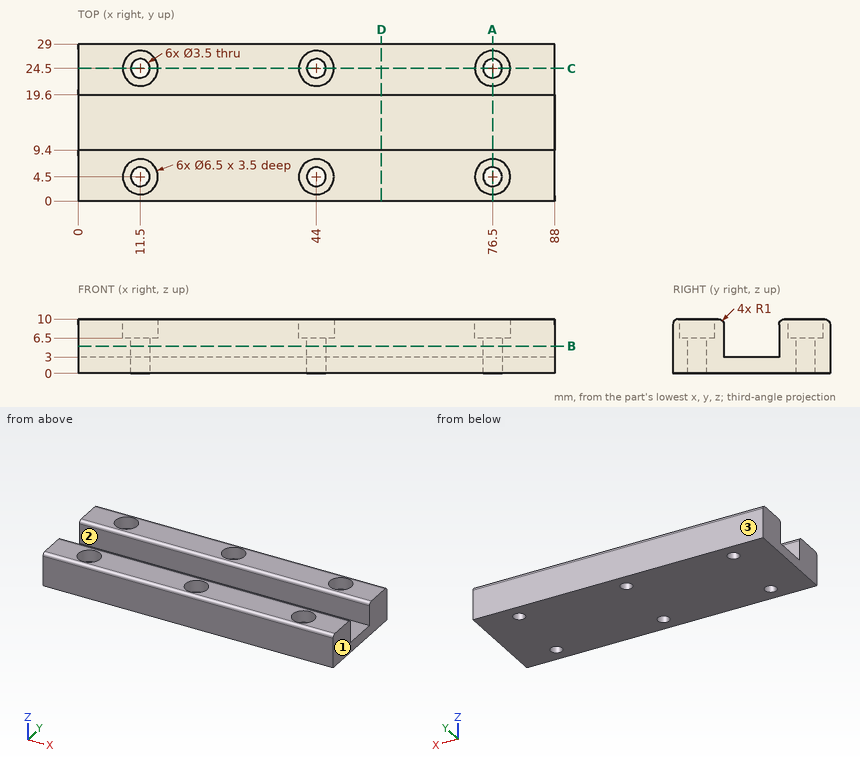
Verification items for this drawing (mm, ordinates from the low corner). Coordinates: 2 decimals unless noted, no trailing zeros. Write each loop counter-clockwise with the first axis right and the second up, starting at its lowest first coordinate (ties: lowest second). Pieces come first, ordered by that corner, then holes. Notation, with made-up numbers: M 6.25,14.5 L 32.25,14.5 A37 cw 32.25,53.5 Z; hole C 78.5,67.5 d3. An arc over 180 degrees is marked long. Use one line per item in the form item = value. Start each with the question number.
1) Thickness scan on probe 1 along Y at (x, z) = (11.5, 8.65); probe 2 along Y at (x, z) = (11.5, 2.75); probe 3 along Y at (x, z) = (76.5, 3.25). Record the ranges inside material, lowest first. Write a range as from..to.
2) Section check B-B on z = 5. Enter the section's corners in (x, y).
3) Release check for a two-part mould opening along Y. For the marked faces 1, 2 and 3 record: pulls with the +Y half, pulls with the -Y half, needs draft (parallel to the pull), parting line crosses it, or undercut.
4) Section check D-D on x = 56. Enter the section's corners in (y, z).
5) Go/stop test with flat-tipped pins: pin 1 Ø2 at (x, y) = (10.5, 23.5) entering from +Z; pin 2 Ø1 at (x, y) = (59.5, 11) entering from +Z. Record where each tip stops, or that it passes through.
6) Section check A-A on x = 76.5. Enter the section's corners in (y, z), and give its area (3 significant figures).
7) Section check C-C on y = 24.5. Enter the section's corners in (x, z).
Responses:
q1.probe_1 = 0..1.25, 7.75..9.4, 19.6..21.25, 27.75..29
q1.probe_2 = 0..2.75, 6.25..22.75, 26.25..29
q1.probe_3 = 0..2.75, 6.25..9.4, 19.6..22.75, 26.25..29
q2.outline = M 0,0 L 88,0 L 88,9.4 L 0,9.4 Z; M 0,19.6 L 88,19.6 L 88,29 L 0,29 Z; hole C 11.5,4.5 d3.5; hole C 11.5,24.5 d3.5; hole C 44,4.5 d3.5; hole C 44,24.5 d3.5; hole C 76.5,4.5 d3.5; hole C 76.5,24.5 d3.5
q3.face_1 = needs draft
q3.face_2 = undercut
q3.face_3 = pulls with the +Y half
q4.outline = M 0,0 L 29,0 L 29,9 A1 ccw 28,10 L 20.6,10 A1 ccw 19.6,9 L 19.6,3 L 9.4,3 L 9.4,9 A1 ccw 8.4,10 L 1,10 A1 ccw 0,9 Z
q5.pin_1 = 6.5
q5.pin_2 = 3
q6.outline = M 0,0 L 2.75,0 L 2.75,6.5 L 1.25,6.5 L 1.25,10 L 1,10 A1 ccw 0,9 Z; M 6.25,0 L 22.75,0 L 22.75,6.5 L 21.25,6.5 L 21.25,10 L 20.6,10 A1 ccw 19.6,9 L 19.6,3 L 9.4,3 L 9.4,9 A1 ccw 8.4,10 L 7.75,10 L 7.75,6.5 L 6.25,6.5 Z; M 26.25,0 L 29,0 L 29,9 A1 ccw 28,10 L 27.75,10 L 27.75,6.5 L 26.25,6.5 Z
q6.area = 127 mm2
q7.outline = M 0,0 L 9.75,0 L 9.75,6.5 L 8.25,6.5 L 8.25,10 L 0,10 Z; M 13.25,0 L 42.25,0 L 42.25,6.5 L 40.75,6.5 L 40.75,10 L 14.75,10 L 14.75,6.5 L 13.25,6.5 Z; M 45.75,0 L 74.75,0 L 74.75,6.5 L 73.25,6.5 L 73.25,10 L 47.25,10 L 47.25,6.5 L 45.75,6.5 Z; M 78.25,0 L 88,0 L 88,10 L 79.75,10 L 79.75,6.5 L 78.25,6.5 Z
